Input: dimensioned drawing with shaded views. Units: mm. Origin: part minimum x, y, z. Coordinates: 2 decimals unless noted, no trailing zeros. One line per question, with ' | ' between items. Start each with the question number.
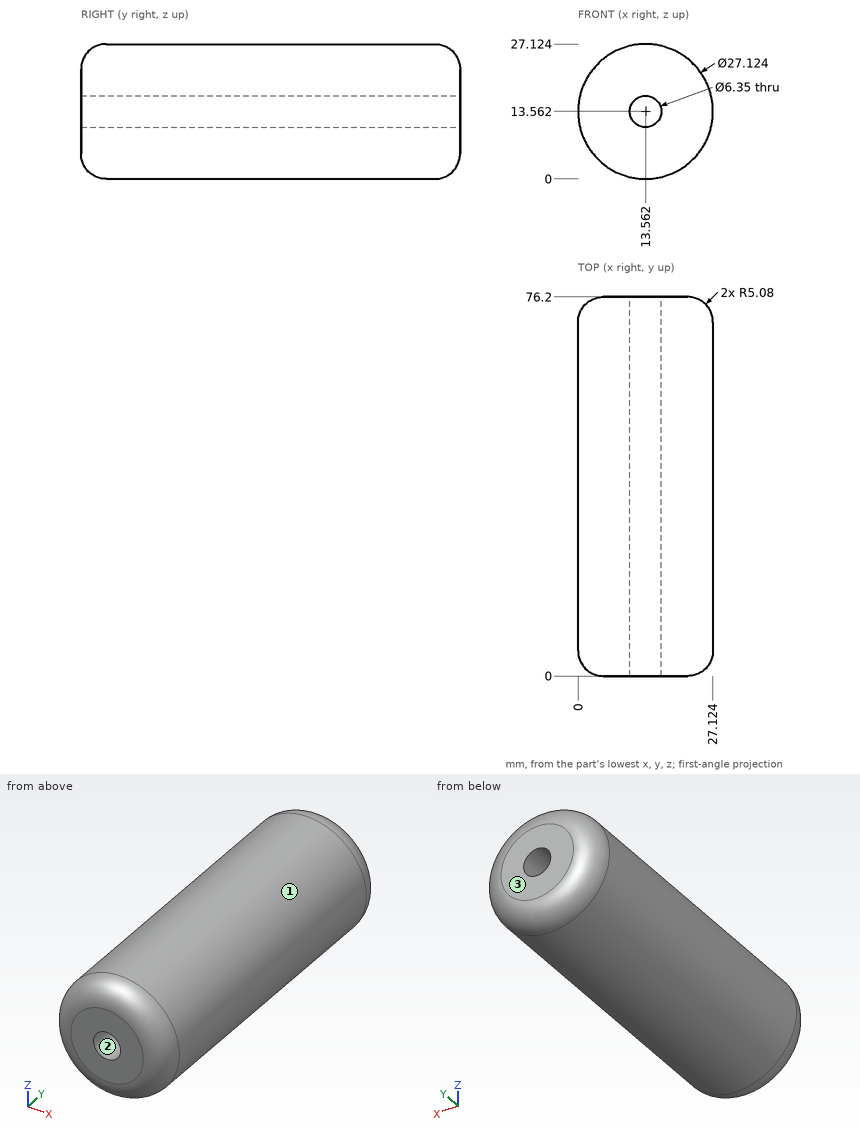
(1) Pin query (flat end, axial travel): pin 1 (10 mm diameter, centred on x = 9, y = 16, fed in from -Z); pin 2 (2 mm diameter, centred on x = 7, y = 55, fed in from +Z); pin 3 (2 mm diameter, centred on y = 10.5, z = 4, fed in from +X); pin 4 (3 mm diameter, centred on x = 9.5, z = 23.5, fed in from +Y). Return the tip coordinate at first contact, or that it passes through.
(2) Draft query along X for the marked faces 1, 2 and 3. Return one class per face: +X half, -X half, draft (parallel to the pull), parting line (faces both ways), or undercut.
(3) Material intervals for line 1 along X through (y, z) = (45, 13.5) (1 decimal); line 2 along X through (y, z) = (9.5, 12) (1 decimal); line 3 along X through (y, z) = (5, 20.75), sorted ascending. Write a range as from..to.
Worked answers:
1) pin 1: stops at z = 0 | pin 2: stops at z = 25.93 | pin 3: stops at x = 24.08 | pin 4: stops at y = 76.14
2) face 1: parting line | face 2: undercut | face 3: draft
3) line 1: x = 0..10.4, 16.7..27.1 | line 2: x = 0.1..10.8, 16.3..27 | line 3: x = 2.06..25.06
